Could you check a few things on this model? Use its own coordinates, in mm. A direction names the side the tool comes from. Coordinates: 2 decimals unless noted, no trailing zeros. Order: outer loops, then holes, each group sorted by start corner. A loop starts at its lowest first (then second) coordinate and runs counter-clockwise, first axis right, second up. Notation, with made-up numbers: (-9.5, 31.25) - (-0.5, 31.25) arc R17 ccw to (-0.5, 56.25) - close; hole circle Ø4 at (47.5, 54). An arc over 180 degrees is marked (long way). Answer as a JSON object with one key per item and string values. Group by question number.
(1) Please list where these lines run through material, in increasing order: probe 1 along X at (y, z) = (27, 7.5); probe 2 along X at (y, z) = (27, 0.9); probe 3 along X at (y, z) = (11, 7.25).
(2) Imagine slicing it at C-C, the plane y = -20. Write out the boundary of the cut face in (x, z).
(3) Imagine slicing it at B-B, the plane y = 7.5. Write out the boundary of the cut face in (x, z).
(4) Imagine slicing it at A-A, the plane x = 25. Write out the boundary of the cut face in (y, z), and give its area (3 significant figures).
(5) We'd pull the mould along X, two halves only. Please class faces 1 (the flat face through (38, 27, 3.5)), 2 (the flat face through (-9, 0, 11)), 3 (the flat face through (45, -21, 5)): pulls with the +X half, pulls with the -X half, needs draft (parallel to the pull), parting line crosses it, or undercut.
(6) Imagine slicing it at D-D, the plane z = 10.25. Give the number of separate pieces and of enclosed holes in the cut face, and give its area (3 significant figures).
(7) Will these pins go through, and if not, where does the flat tip stop? P1, Ø2, axis at y = 4.5, z = 1, coming from the +X side; P2, Ø1, axis at y = 5.5, z = 4, coming from the +X side; P3, Ø1.7, axis at x = 36, y = -12, coming from the -Z side.
(8) Which directions (+Z, -Z, +X, -X, +Y, -Y) give clear straight access to the entire face, cutting with the end or side of a thin tool? Please do faces 4 (the cylindrical face through (27.146, 8.176, 0.986)), 5 (the flat face through (-6, 29, 3.5)), 6 (the cylindrical face through (36.6, -19.9, 6.9)).
from build123d import *

# Parameters (mm, degrees)
SKETCH_W                       = 55
SKETCH_H                       = 60
PAD_DEPTH                      = 11
SKETCH001_R                    = 7.6
POCKET_DEPTH                   = 60.001
SKETCH002_R                    = 1.75
POCKET001_DEPTH                = 11.001
POCKET002_DEPTH                = 9
SKETCH004_R                    = 2.25
POCKET003_DEPTH                = 11.001
SKETCH008_R                    = 4.1
POCKET005_DEPTH                = 20
SKETCH010_W                    = 20
SKETCH010_H                    = 25
POCKET006_DEPTH                = 5
CHAMFER_SIZE                   = 3
CHAMFER001_SIZE                = 3
PART_MIRRORING_PLACEMENT_ANGLE = 180
SKETCH011_R                    = 2.9
POCKET007_DEPTH                = 3.5


with BuildPart() as chamfer002:
    # Sketch → Pad (new body)
    with BuildSketch(Plane.XY):
        with Locations((17.5, 0)):
            Rectangle(SKETCH_W, SKETCH_H)
    extrude(amount=PAD_DEPTH)

    # Sketch001 → Pocket (cut, through all)
    with BuildSketch(Plane.XZ.offset(30)):
        with Locations((0, 11)):
            Circle(SKETCH001_R)
    extrude(amount=-POCKET_DEPTH, mode=Mode.SUBTRACT)

    # Sketch002 → Pocket001 (cut, through all)
    with BuildSketch(Plane(origin=(0, 0, 0), x_dir=(1, 0, 0), z_dir=(0, 0, -1))):
        with Locations((-6, 27)):
            Circle(SKETCH002_R)
        with Locations((36, 27)):
            Circle(SKETCH002_R)
        with Locations((-6, -27)):
            Circle(SKETCH002_R)
        with Locations((36, -27)):
            Circle(SKETCH002_R)
        with Locations((6, 27)):
            Circle(SKETCH002_R)
        with Locations((6, -27)):
            Circle(SKETCH002_R)
        with Locations((6, 0)):
            Circle(SKETCH002_R)
        with Locations((-6, 0)):
            Circle(SKETCH002_R)
        with Locations((36, -13)):
            Circle(SKETCH002_R)
        with Locations((36, 13)):
            Circle(SKETCH002_R)
    extrude(amount=-POCKET001_DEPTH, mode=Mode.SUBTRACT)

    # Sketch003 → Pocket002 (cut)
    with BuildSketch(Plane.XY.offset(11)):
        with BuildLine():
            Line((10, 35), (10, -35))
            Line((10, -35), (28, -35))
            Line((28, -35), (28, -14.916198))
            ThreePointArc((28, -14.916198), (30.841983, -12.965458), (32.599342, -10))
            Line((32.599342, -10), (52.599342, -10))
            Line((52.599342, -10), (52.599342, 10))
            Line((52.599342, 10), (32.599342, 10))
            ThreePointArc((32.599342, 10), (30.841983, 12.965458), (28, 14.916198))
            Line((28, 14.916198), (28, 35))
            Line((28, 35), (10, 35))
        make_face()
    extrude(amount=-POCKET002_DEPTH, mode=Mode.SUBTRACT)

    # Sketch004 → Pocket003 (cut, through all)
    with BuildSketch(Plane(origin=(0, 0, 0), x_dir=(1, 0, 0), z_dir=(0, 0, -1))):
        with Locations((25, 7.5)):
            Circle(SKETCH004_R)
        with Locations((25, -7.5)):
            Circle(SKETCH004_R)
    extrude(amount=-POCKET003_DEPTH, mode=Mode.SUBTRACT)

    # Sketch008 → Pocket005 (cut)
    with BuildSketch(Plane.YZ.offset(45)):
        with Locations((-20, 11)):
            Circle(SKETCH008_R)
        with Locations((20, 11)):
            Circle(SKETCH008_R)
    extrude(amount=-POCKET005_DEPTH, mode=Mode.SUBTRACT)

    # Sketch010 → Pocket006 (cut)
    with BuildSketch(Plane.YZ.offset(45)):
        with Locations((0, 3.5)):
            Rectangle(SKETCH010_W, SKETCH010_H)
    extrude(amount=-POCKET006_DEPTH, mode=Mode.SUBTRACT)

    # Chamfer
    chamfer_edges = [chamfer002.edges().sort_by_distance(p)[0] for p in [
        (45, -10, 6.5),
    ]]
    chamfer(chamfer_edges, length=CHAMFER_SIZE)

    # Chamfer001
    chamfer001_edges = [chamfer002.edges().sort_by_distance(p)[0] for p in [
        (45, 10, 6.5),
    ]]
    chamfer(chamfer001_edges, length=CHAMFER001_SIZE)


with BuildPart() as pocket007:
    # Part__Mirroring: instance of Chamfer002
    add(chamfer002.part.mirror(Plane(origin=(0, 0, 0), x_dir=(0, 1, 0), z_dir=(0, 0, 1))))


with BuildPart() as pocket007_1:
    # Part__Mirroring placement: moved
    add(pocket007.part.rotate(Axis((0, 0, 0), (1, 0, 0)), PART_MIRRORING_PLACEMENT_ANGLE))

    # Sketch011 → Pocket007 (cut)
    with BuildSketch(Plane(origin=(0, 0, 0), x_dir=(1, 0, 0), z_dir=(0, 0, -1))):
        with Locations((36, 27)):
            Circle(SKETCH011_R)
        with Locations((36, 13)):
            Circle(SKETCH011_R)
        with Locations((36, -13)):
            Circle(SKETCH011_R)
        with Locations((36, -27)):
            Circle(SKETCH011_R)
        with Locations((-6, 27)):
            Circle(SKETCH011_R)
        with Locations((6, 27)):
            Circle(SKETCH011_R)
        with Locations((-6, 0)):
            Circle(SKETCH011_R)
        with Locations((6, 0)):
            Circle(SKETCH011_R)
        with Locations((-6, -27)):
            Circle(SKETCH011_R)
        with Locations((6, -27)):
            Circle(SKETCH011_R)
    extrude(amount=-POCKET007_DEPTH, mode=Mode.SUBTRACT)


solid = pocket007_1.part
Result set:
{
 "1": {"probe 1": "x = -10 to -7.75, 7.75 to 10, 28 to 34.25, 37.75 to 45", "probe 2": "x = -10 to -8.9, -3.1 to 3.1, 8.9 to 33.1, 38.9 to 45", "probe 3": "x = -10 to -6.61, 6.61 to 10, 32.19 to 43"},
 "2": {"outline": "(-10, 0) - (45, 0) - (45, 6.9) - (28, 6.9) - (28, 2) - (10, 2) - (10, 11) - (7.6, 11) arc R7.6 cw to (-7.6, 11) - (-10, 11) - close"},
 "3": {"outline": "(-10, 0) - (22.75, 0) - (22.75, 2) - (10, 2) - (10, 11) - (7.6, 11) arc R7.6 cw to (-7.6, 11) - (-10, 11) - close; (27.25, 0) - (40, 0) - (40, 2) - (27.25, 2) - close"},
 "4": {"outline": "(-30, 0) - (-9.75, 0) - (-9.75, 2) - (-30, 2) - close; (-5.25, 0) - (5.25, 0) - (5.25, 2) - (-5.25, 2) - close; (9.75, 0) - (30, 0) - (30, 2) - (9.75, 2) - close", "area": "102 mm^2"},
 "5": {"face 1": "undercut", "face 2": "needs draft", "face 3": "pulls with the +X half"},
 "6": {"separate pieces": "6", "enclosed holes": "4", "area": "620 mm^2"},
 "7": {"P1": "stops at x = 40", "P2": "stops at x = 10", "P3": "stops at z = 3.5"},
 "8": {"face 4": "+Z, -Z", "face 5": "-Z", "face 6": "+Z, +X"}
}
